Job drawing, mm, ordinate dimensions from the low corner. One solid piece. Round coordinates to 2 decimals unless told otherwise and drop trailing zeros. Loops run counter-clockwise (first coordinate to the right, second up) from the corner with the lowest first, then second, coordinate; pieces in that order, holes last.
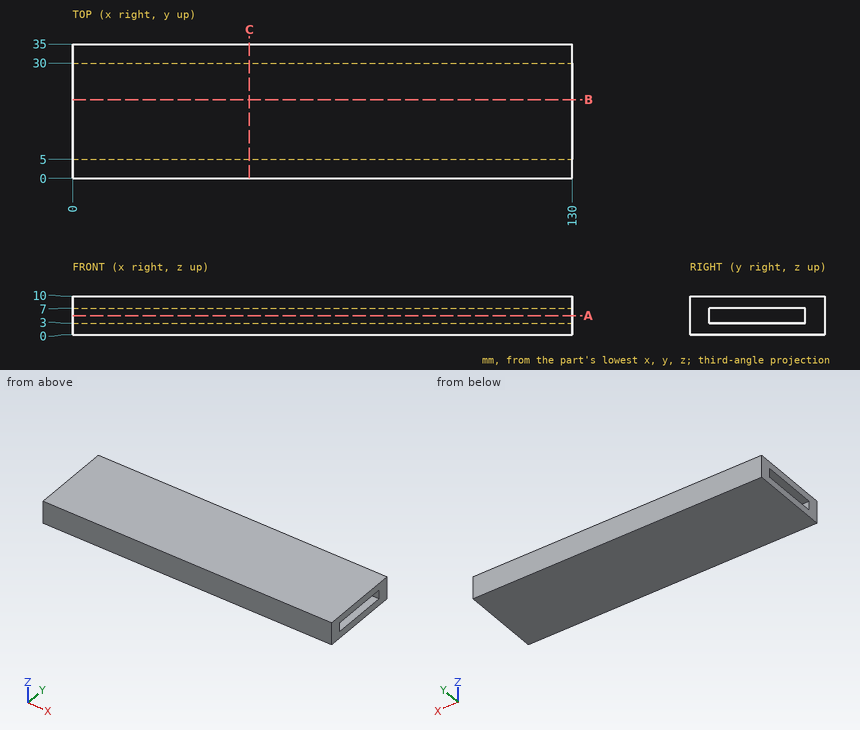
1) Slice it at B-B, the plane y = 20.5. Give the cut face in (x, z).
Values:
outline: (0, 0) - (130, 0) - (130, 3) - (0, 3) - close; (0, 7) - (130, 7) - (130, 10) - (0, 10) - close
2) Slice it at A-A, the plane z = 5. Give the cut face in (x, y).
Values:
outline: (0, 0) - (130, 0) - (130, 5) - (0, 5) - close; (0, 30) - (130, 30) - (130, 35) - (0, 35) - close
3) Wall check: line 1 along Z through (x, y) = (19, 21.5); line 2 along Y through (x, z) = (60, 3.25). Give the ranges that are in metal, low to high.
Values:
line 1: z = 0 to 3, 7 to 10
line 2: y = 0 to 5, 30 to 35
4) Slice it at C-C, the plane x = 46. Give the cut face in (y, z), then the cut area to 3 significant figures.
Values:
outline: (0, 0) - (35, 0) - (35, 10) - (0, 10) - close; hole (5, 3) - (30, 3) - (30, 7) - (5, 7) - close
area: 250 mm2
5) Drop a flat-ended pin along its axis: pin 1 Ø8 at (x, y) = (22, 10) entering from -Z. Give the stop position or say it passes through.
Values:
pin 1: stops at z = 0
